Verification items for the finished model (mm, model axes). A direction names the side the tool comes from. Round coordinates to 2 decimals unless told otherwise and drop trailing zeros. Loops run counter-clockwise (first coordinate to the right, second up) from the corner with the lowest first, then second, coordinate; pieces in that order, holes last. Notation, with made-up numbers: (11, -25.5) - (44, -25.5) arc R28 cw to (44, -3.5) - close; hole circle Ø5 at (54.25, -19). An arc over 180 degrees is marked (long way). Use CSV: the item, a comma, the result in double quotes.
```python
from build123d import *

# Parameters (mm, degrees)
BOSS_EXTRUDE1_DEPTH = 3
SKETCH3_R           = 1.375
CUT_EXTRUDE1_DEPTH  = 4
FILLET1_R           = 8


with BuildPart() as part:
    # Sketch2 → Boss-Extrude1 (new body)
    with BuildSketch(Plane(origin=(0, 0, 0), x_dir=(1, 0, 0), z_dir=(0, 1, 0))):
        with BuildLine():
            Line((-12.66542378, 21.955324516), (-12.66542378, 15.25))
            ThreePointArc((-12.66542378, 15.25), (-12.810144222, 14.202492305), (-13.233463188, 13.233463188))
            Line((-13.233463188, 13.233463188), (-22.5, 0))
            Line((-22.5, 0), (-24.625, 0))
            ThreePointArc((-24.625, 0), (-26, 1.375), (-27.375, 0))
            Line((-27.375, 0), (-28.75, 0))
            ThreePointArc((-28.75, 0), (-28.622713939, 0.826965294), (-28.252638839, 1.57737702))
            Line((-28.252638839, 1.57737702), (-17.83457622, 16.455324516))
            Line((-17.83457622, 16.455324516), (-17.83457622, 21.955324516))
            ThreePointArc((-17.83457622, 21.955324516), (-15.25, 24.539900736), (-12.66542378, 21.955324516))
        make_face()
    boss_extrude1 = extrude(amount=BOSS_EXTRUDE1_DEPTH)

    # Sketch3 → Cut-Extrude1 (cut, through all)
    with BuildSketch(Plane(origin=(0, 3, 0), x_dir=(1, 0, 0), z_dir=(0, 1, 0))):
        with Locations((-15.25, 15.25)):
            Circle(SKETCH3_R)
        with Locations((-15.25, 21.955324516)):
            Circle(SKETCH3_R)
    cut_extrude1 = extrude(amount=-CUT_EXTRUDE1_DEPTH, mode=Mode.SUBTRACT)

    # Mirror2: Boss-Extrude1, Cut-Extrude1 across plane
    add(boss_extrude1.mirror(Plane(origin=(-22.5, 3, 0), x_dir=(1, 0, 0), z_dir=(0, 0, -1))))
    add(cut_extrude1.mirror(Plane(origin=(-22.5, 3, 0), x_dir=(1, 0, 0), z_dir=(0, 0, -1))), mode=Mode.SUBTRACT)

    # Fillet1
    fillet1_edges = [part.edges().sort_by_distance(p)[0] for p in [
        (-17.83457622, 1.5, -16.455324516),
        (-22.5, 1.5, 0),
        (-17.83457622, 1.5, 16.455324516),
    ]]
    fillet(fillet1_edges, radius=FILLET1_R)


solid = part.part
```
1) Cross-section at A-A, the plane y = 2.5. Record the cut outline in (x, z) (3 decimals), then the cut area to 3 significant figures.
Returned:
outline,"(-28.253, -1.577) - (-19.281, -14.389) arc R8 cw to (-17.835, -18.978) - (-17.835, -21.955) arc R2.585 ccw to (-12.665, -21.955) - (-12.665, -15.25) arc R3.863 ccw to (-13.233, -13.233) - (-19.287, -4.589) arc R8 cw to (-19.287, 4.589) - (-13.233, 13.233) arc R3.863 ccw to (-12.665, 15.25) - (-12.665, 21.955) arc R2.585 ccw to (-17.835, 21.955) - (-17.835, 18.978) arc R8 cw to (-19.281, 14.389) - (-28.253, 1.577) arc R2.75 ccw to start; hole circle Ø2.75 at (-26, 0); hole circle Ø2.75 at (-15.25, -21.955); hole circle Ø2.75 at (-15.25, -15.25); hole circle Ø2.75 at (-15.25, 15.25); hole circle Ø2.75 at (-15.25, 21.955)"
area,"276 mm²"
2) Thickness scan on probe 1 along Z at (x, y) = (-15.25, 0.85) (3 decimals); probe 2 along Z at (x, y) = (-15, 1.15); probe 3 along X at (y, z) = (1.55, 15.25) (3 decimals). Record the ranges inside material, lowest first. Write a range as [from, to].
Returned:
probe 1,"z = [-24.54, -23.33], [-20.58, -16.625], [-13.875, -10.354], [10.354, 13.875], [16.625, 20.58], [23.33, 24.54]"
probe 2,"z = [-24.53, -23.31], [-20.6, -16.6], [-13.9, -10.71], [10.71, 13.9], [16.6, 20.6], [23.31, 24.53]"
probe 3,"x = [-18.756, -16.625], [-13.875, -12.665]"
3) Cross-section at C-C, the plane x = -15.25. Record the cut outline in (y, z) (3 decimals).
Returned:
outline,"(0, -24.54) - (3, -24.54) - (3, -23.33) - (0, -23.33) - close; (0, -20.58) - (3, -20.58) - (3, -16.625) - (0, -16.625) - close; (0, -13.875) - (3, -13.875) - (3, -10.354) - (0, -10.354) - close; (0, 10.354) - (3, 10.354) - (3, 13.875) - (0, 13.875) - close; (0, 16.625) - (3, 16.625) - (3, 20.58) - (0, 20.58) - close; (0, 23.33) - (3, 23.33) - (3, 24.54) - (0, 24.54) - close"
4) Cross-section at D-D, the plane x = -18.5. Record the cut outline in (y, z), then the cut area to 3 significant figures.
Returned:
outline,"(0, -15.78) - (3, -15.78) - (3, -5.71) - (0, -5.71) - close; (0, 5.71) - (3, 5.71) - (3, 15.78) - (0, 15.78) - close"
area,"60.4 mm²"
5) Cross-section at B-B, the plane x = -26. Record the cut outline in (y, z) (3 decimals), then the cut area to 3 significant figures.
Returned:
outline,"(0, -4.794) - (3, -4.794) - (3, -1.375) - (0, -1.375) - close; (0, 1.375) - (3, 1.375) - (3, 4.794) - (0, 4.794) - close"
area,"20.5 mm²"
6) Gauge pin test, flat ends, axial feed: pin 1 Ø1 at (y, z) = (2, -15) entering from -X; pin 2 Ø1.5 at (y, z) = (1.5, 20) entering from -X. Record the tip position at first contact, or that the pin passes through.
Returned:
pin 1,"stops at x = -19.21"
pin 2,"stops at x = -17.83"
7) Mould release check, pull along Z, two halves, no side actions. Record for faces 4 (the face through (-12.806, 1.479, 14.217)), 5 (the face through (-21, 0, -2)), 6 (the face through (-18.215, 1.521, -16.539)), 7 (the face through (-16.2, 1.5, -9)): +Z half, -Z half, draft (parallel to the pull), parting line (faces both ways), or undercut.
Returned:
face 4,"undercut"
face 5,"draft"
face 6,"-Z half"
face 7,"undercut"
8) Access from +Z, -Z, +X, -X, +Y, -Y to the whole of each face (thin tool, end or side, straight path). Record for faces 1 (the face through (-12.806, 1.479, -14.217)), 2 (the face through (-16.624, 1.521, -22.016)), 3 (the face through (-17.835, 1, 20)).
Returned:
face 1,"+X, +Y, -Y"
face 2,"+Y, -Y"
face 3,"+Z, -X, +Y, -Y"
